from build123d import *

# Parameters (mm, degrees)
PAD_DEPTH    = 6
SKETCH001_R  = 6
PAD001_DEPTH = 20
SKETCH002_R  = 1.7
POCKET_DEPTH = 6.001
FILLET_R     = 5


with BuildPart() as part:
    # Sketch → Pad (new body)
    with BuildSketch(Plane.XY):
        with BuildLine():
            ThreePointArc((-15.905974, 6), (0, -17), (15.905974, 6))
            Line((-15.905974, 6), (15.905974, 6))
        make_face()
    extrude(amount=PAD_DEPTH)

    # Sketch001 → Pad001 (new body)
    with BuildSketch(Plane(origin=(0, 0, 0), x_dir=(1, 0, 0), z_dir=(0, 0, -1))):
        Circle(SKETCH001_R)
    extrude(amount=PAD001_DEPTH)

    # Sketch002 → Pocket (cut, through all)
    with BuildSketch(Plane(origin=(0, 0, 0), x_dir=(1, 0, 0), z_dir=(0, 0, -1))):
        with Locations((12, 0)):
            Circle(SKETCH002_R)
        with Locations((-12, 0)):
            Circle(SKETCH002_R)
        with Locations((0, 12)):
            Circle(SKETCH002_R)
    extrude(amount=-POCKET_DEPTH, mode=Mode.SUBTRACT)

    # Fillet
    fillet_edges = [part.edges().sort_by_distance(p)[0] for p in [
        (-15.905974, 6, 3),
        (15.905974, 6, 3),
    ]]
    fillet(fillet_edges, radius=FILLET_R)


solid = part.part
Geometry: final body of the model. Coordinates: model frame, mm. A direction names the side the tool comes from. Coordinates: 2 decimals unless noted, no trailing zeros. Order: outer loops, then holes, each group sorted by start corner. A loop starts at its lowest first (then second) coordinate and runs counter-clockwise, first axis right, second up.
1) Section C-C (y = 0). Return loops of the section in (x, z).
Result sheet:
outline: (-17, 0) - (-13.7, 0) - (-13.7, 6) - (-17, 6) - close; (-10.3, 0) - (-6, 0) - (-6, -20) - (6, -20) - (6, 0) - (10.3, 0) - (10.3, 6) - (-10.3, 6) - close; (13.7, 0) - (17, 0) - (17, 6) - (13.7, 6) - close
2) Section D-D (x = -3). Return loops of the section in (y, z), then the cut area to 3 significant figures.
Result sheet:
outline: (-16.73, 0) - (-5.2, 0) - (-5.2, -20) - (5.2, -20) - (5.2, 0) - (6, 0) - (6, 6) - (-16.73, 6) - close
area: 344 mm2
3) Section A-A (z = 0.5). Return loops of the section in (x, y), then the cut area to 3 significant figures.
Result sheet:
outline: (-16.94, 1.42) arc R17 ccw (long way) to (16.94, 1.42) arc R5 ccw to (11.96, 6) - (-11.96, 6) arc R5 ccw to start; hole circle Ø3.4 at (-12, 0); hole circle Ø3.4 at (0, -12); hole circle Ø3.4 at (12, 0)
area: 620 mm2
4) Draft query along X for faces 1 (the cylindrical face through (-0.221, -13.686, 2.958)), 2 (the cylindrical face through (0, -17, 3)), 3 (the flat face through (0, -3, 6)). Return one class per face: released by +X, released by -X, zero draft, split by the parting line, or undercut.
Result sheet:
face 1: undercut
face 2: split by the parting line
face 3: zero draft
5) Section B-B (y = -12). Return loops of the section in (x, z), then the cut area to 3 significant figures.
Result sheet:
outline: (-12.04, 0) - (-1.7, 0) - (-1.7, 6) - (-12.04, 6) - close; (1.7, 0) - (12.04, 0) - (12.04, 6) - (1.7, 6) - close
area: 124 mm2
6) Set-up query: faces 4 (the cylindrical face through (-6, 0, -10)), 5 (the flat face through (0, 0, -20)). Return all of +Z, -Z, +X, -X, +Y, -Y with unobstructed straight access to the full face (end or side cutting, diameter ignored); none if empty.
Result sheet:
face 4: -Z
face 5: -Z, +X, -X, +Y, -Y
7) First-contact query: P1, Ø4, axis at x = 8, y = -14, coming from the -Z side; P2, Ø6, axis at y = 0.5, z = -15, coming from the -X side; P3, Ø1, axis at y = -1.5, z = -13.5, coming from the -X side; P4, Ø3, axis at x = 12, y = 0, coming from the -Z side. Flat tips, straight axial feed; report the tip coordinate or a pass-through.
Result sheet:
P1: stops at z = 0
P2: stops at x = -6
P3: stops at x = -5.92
P4: passes through
8) Ray query, probe 1 along X at (y, z) = (0, 3.05); probe 2 along Z at (x, y) = (-7.5, -7); probe 3 along Y at (x, z) = (12, 2.6). Return the intervals inside material, ascending.
Result sheet:
probe 1: x = -17 to -13.7, -10.3 to 10.3, 13.7 to 17
probe 2: z = 0 to 6
probe 3: y = -12.04 to -1.7, 1.7 to 6
